```python
from build123d import *

# Parameters (mm, degrees)
F0_R     = 1.7
F1_DEPTH = 5
F2_DEPTH = 30
F3_DEPTH = 20
F4_W     = 7.581357
F4_H     = 5
F5_DEPTH = 50.001
F6_SIZE  = 3


with BuildPart() as f1:
    # F0 (on Top) → F1 (new body)
    with BuildSketch(Plane.XY):
        Polygon((29.865686, -22.586415), (21.444556, -22.586415), (21.444556, -47.586415), (21.444556, -72.586415), (29.865686, -72.586415), (29.865686, -57.586415), (29.865686, -47.586415), (29.865686, -37.586415), align=None)
        with Locations((26.444556, -67.586415)):
            Circle(F0_R, mode=Mode.SUBTRACT)
        with Locations((26.444556, -27.586415)):
            Circle(F0_R, mode=Mode.SUBTRACT)
        Polygon((49.868173, -22.586415), (41.447043, -22.586415), (41.447043, -37.586415), (41.447043, -47.586415), (41.447043, -57.586415), (41.447043, -72.586415), (49.868173, -72.586415), (49.868173, -47.586415), align=None)
        with Locations((44.868173, -67.586415)):
            Circle(F0_R, mode=Mode.SUBTRACT)
        with Locations((44.868173, -27.586415)):
            Circle(F0_R, mode=Mode.SUBTRACT)
    extrude(amount=F1_DEPTH)

    # F0 (on Top) → F2 (join)
    with BuildSketch(Plane.XY):
        Polygon((35.656365, -22.586415), (29.865686, -22.586415), (29.865686, -37.586415), (35.656365, -37.586415), (41.447043, -37.586415), (41.447043, -22.586415), align=None)
        Polygon((29.865686, -57.586415), (29.865686, -72.586415), (35.656365, -72.586415), (41.447043, -72.586415), (41.447043, -57.586415), (35.656365, -57.586415), align=None)
    extrude(amount=F2_DEPTH)

    # F0 (on Top) → F3 (join)
    with BuildSketch(Plane.XY):
        Polygon((35.656365, -37.586415), (29.865686, -37.586415), (29.865686, -47.586415), (29.865686, -57.586415), (35.656365, -57.586415), (41.447043, -57.586415), (41.447043, -47.586415), (41.447043, -37.586415), align=None)
    extrude(amount=F3_DEPTH)

    # F4 (on face) → F5 (cut, through all)
    with BuildSketch(Plane.XZ.offset(72.586415)):
        with Locations((35.656365, 24.5)):
            Rectangle(F4_W, F4_H)
    extrude(amount=-F5_DEPTH, mode=Mode.SUBTRACT)

    # F6
    f6_edges = [f1.edges().sort_by_distance(p)[0] for p in [
        (31.865686, -30.086415, 27),
        (31.865686, -65.086415, 27),
        (39.447043, -30.086415, 27),
        (39.447043, -65.086415, 27),
    ]]
    chamfer(f6_edges, length=F6_SIZE)


solid = f1.part
```
The model under review builds one solid part; all positions refer to its coordinate system, in mm. A direction names the side the tool comes from. Coordinates: 2 decimals unless noted, no trailing zeros. Order: outer loops, then holes, each group sorted by start corner. A loop starts at its lowest first (then second) coordinate and runs counter-clockwise, first axis right, second up. Notation, with made-up numbers: (54, 58.5) -> (62, 58.5) arc R20 ccw to (62, 74.5) -> close; hole circle Ø10 at (35.5, 61). An arc over 180 degrees is marked (long way). Answer in a Markdown table with one row per item. Add a question column.
Item 1: Machinability: for faces 5 (the flat face through (36, -30, 22)), 6 (the flat face through (46, -47, 5)), 7 (the flat face through (36, -65, 30)), which of the approach directions +Z, -Z, +X, -X, +Y, -Y give a long, thin tool a straight path to every point of the face, cutting with its end or side? Answer none if there is none.
Item 2: To check wall thickness, follow probe 1 along X at (y, z) = (-67, 3.25); probe 2 along Y at (x, z) = (36.25, 28); probe 3 along Z at (x, y) = (41.75, -29). State the ranges of each line that lie inside material, in increasing order.
Item 3: We need section C-C on x = 37. Write out the cut boundary in (y, z), plus the area to 3 significant figures.
Item 4: We need section B-B on y = -33. Write out the cut boundary in (x, z).
Item 5: We need section A-A on z = 22.75. Write out the cut boundary in (x, y), plus the area to 3 significant figures.
Item 6: Mouldability with a two-part tool opening along X and no side actions: class faces 1 (the flat face through (26, -47, 5)), 2 (the flat face through (29.866, -47, 17)), 3 (the flat face through (49.868, -48, 2)), 4 (the flat face through (39.447, -30, 23)) as +X half, -X half, draft (parallel to the pull), parting line (faces both ways), or undercut.
Item 7: We need section D-D on x = 40. Write out the cut boundary in (y, z), plus the area to 3 significant figures.
Item 8: Clearance check with flat-ended pins moving along their axes: pin 1 (2 mm diameter, centred on y = -37, z = 12, fed in from +X); pin 2 (1.6 mm diameter, centred on y = -66.5, z = 23, fed in from -X); pin 3 (3.5 mm diameter, centred on x = 34, y = -45, fed in from +Z). State where each tip first meets the part, or that it passes through.
Final values:
| question | item | result |
|---|---|---|
| 1 | face 5 | +Y, -Y |
| 1 | face 6 | +Z, +X, +Y, -Y |
| 1 | face 7 | +Z, +X, -X, +Y, -Y |
| 2 | probe 1 | x = 21.44 to 24.85, 28.04 to 43.27, 46.46 to 49.87 |
| 2 | probe 2 | y = -72.59 to -57.59, -37.59 to -22.59 |
| 2 | probe 3 | z = 0 to 5 |
| 3 | outline | (-72.59, 0) -> (-22.59, 0) -> (-22.59, 22) -> (-37.59, 22) -> (-37.59, 20) -> (-57.59, 20) -> (-57.59, 22) -> (-72.59, 22) -> close; (-72.59, 26.45) -> (-57.59, 26.45) -> (-57.59, 30) -> (-72.59, 30) -> close; (-37.59, 26.45) -> (-22.59, 26.45) -> (-22.59, 30) -> (-37.59, 30) -> close |
| 3 | area | 1,170 mm2 |
| 4 | outline | (21.44, 0) -> (49.87, 0) -> (49.87, 5) -> (41.45, 5) -> (41.45, 30) -> (29.87, 30) -> (29.87, 5) -> (21.44, 5) -> close; hole (31.87, 22) -> (39.45, 22) -> (39.45, 24) -> (36.45, 27) -> (34.87, 27) -> (31.87, 24) -> close |
| 5 | outline | (29.87, -72.59) -> (31.87, -72.59) -> (31.87, -57.59) -> (29.87, -57.59) -> close; (29.87, -37.59) -> (31.87, -37.59) -> (31.87, -22.59) -> (29.87, -22.59) -> close; (39.45, -72.59) -> (41.45, -72.59) -> (41.45, -57.59) -> (39.45, -57.59) -> close; (39.45, -37.59) -> (41.45, -37.59) -> (41.45, -22.59) -> (39.45, -22.59) -> close |
| 5 | area | 120 mm2 |
| 6 | face 1 | draft |
| 6 | face 2 | -X half |
| 6 | face 3 | +X half |
| 6 | face 4 | undercut |
| 7 | outline | (-72.59, 0) -> (-22.59, 0) -> (-22.59, 30) -> (-37.59, 30) -> (-37.59, 20) -> (-57.59, 20) -> (-57.59, 30) -> (-72.59, 30) -> close |
| 7 | area | 1,300 mm2 |
| 8 | pin 1 | stops at x = 41.45 |
| 8 | pin 2 | stops at x = 29.87 |
| 8 | pin 3 | stops at z = 20 |
